from build123d import *

# Parameters (mm, degrees)
SKETCH1_W           = 20
SKETCH1_H           = 20
BOSS_EXTRUDE1_DEPTH = 5.4
SKETCH2_R           = 8
CUT_EXTRUDE1_DEPTH  = 5
SKETCH4_W           = 1
SKETCH4_H           = 20
CUT_EXTRUDE3_DEPTH  = 10
SKETCH3_R           = 1.5
CUT_EXTRUDE2_DEPTH  = 0.25
SKETCH5_W           = 5.4
SKETCH5_H           = 1
CUT_EXTRUDE4_DEPTH  = 0.25
FILLET1_R           = 1
CHAMFER1_SIZE       = 0.5


with BuildPart() as part:
    # Sketch1 → Boss-Extrude1 (new body)
    with BuildSketch(Plane.XY):
        Rectangle(SKETCH1_W, SKETCH1_H)
    extrude(amount=BOSS_EXTRUDE1_DEPTH)

    # Sketch2 → Cut-Extrude1 (cut)
    with BuildSketch(Plane.XY.offset(5.4)):
        Circle(SKETCH2_R)
    extrude(amount=-CUT_EXTRUDE1_DEPTH, mode=Mode.SUBTRACT)

    # Sketch4 → Cut-Extrude3 (cut)
    with BuildSketch(Plane.XY.offset(5.4)):
        with Locations((9.5, 0)):
            Rectangle(SKETCH4_W, SKETCH4_H)
    extrude(amount=-CUT_EXTRUDE3_DEPTH, mode=Mode.SUBTRACT)

    # Sketch3 → Cut-Extrude2 (cut)
    with BuildSketch(Plane(origin=(9, 0, 0), x_dir=(0, 0, -1), z_dir=(1, 0, 0))):
        with Locations(Location((-2.7, -5, 0), (0, 0, 90))):
            Circle(SKETCH3_R)
    extrude(amount=-CUT_EXTRUDE2_DEPTH, mode=Mode.SUBTRACT)

    # Sketch5 → Cut-Extrude4 (cut)
    with BuildSketch(Plane.ZY.offset(10)):
        with Locations((2.7, 5)):
            Rectangle(SKETCH5_W, SKETCH5_H)
    extrude(amount=-CUT_EXTRUDE4_DEPTH, mode=Mode.SUBTRACT)

    # Fillet1
    fillet1_edges = [part.edges().sort_by_distance(p)[0] for p in [
        (9, -10, 2.7),
        (9, 10, 2.7),
        (-10, -10, 2.7),
        (-10, 10, 2.7),
    ]]
    fillet(fillet1_edges, radius=FILLET1_R)

    # Chamfer1
    # the kernel refuses this chamfer: 0.5 mm, written as the material it takes off along each edge
    with BuildSketch(Plane(origin=(8, 10, 0), x_dir=(0, -0.9996219169112968, -0.02749587661058639), z_dir=(-1, 0, 0)), Plane(origin=(-9, -10, 5.4), x_dir=(0, -0.027495876610585647, -0.9996219169112968), z_dir=(1, 0, 0))) as chamfer1_piece_1:
        Polygon((CHAMFER1_SIZE * 0.999621916911, CHAMFER1_SIZE * 0.0274958766106), (-CHAMFER1_SIZE * 0.0274958766106, CHAMFER1_SIZE * 0.999621916911), (0, 0), align=None)
    extrude(amount=17, mode=Mode.SUBTRACT)
    with BuildSketch(Plane(origin=(-9, 9, 0), x_dir=(0, 1, 0), z_dir=(1, 0, 0))) as chamfer1_piece_2:
        Polygon((1 - CHAMFER1_SIZE, 0), (1, CHAMFER1_SIZE), (1, 0), align=None)
    revolve(axis=Axis((-9, 9, 0), (0, 0, 1)), revolution_arc=90, mode=Mode.SUBTRACT)
    with BuildSketch(Plane(origin=(-10, 5.785841494, 0), x_dir=(0.9996219169112968, 0, -0.02749587661058639), z_dir=(0, -1, 0))) as chamfer1_piece_3:
        Polygon((CHAMFER1_SIZE * 0.999621916911, CHAMFER1_SIZE * 0.0274958766106), (-CHAMFER1_SIZE * 0.0274958766106, CHAMFER1_SIZE * 0.999621916911), (0, 0), align=None)
    extrude(amount=14.785841494, mode=Mode.SUBTRACT)
    with BuildSketch(Plane(origin=(-10, 9, 0), x_dir=(0.9996219169112968, 0, -0.02749587661058639), z_dir=(0, -1, 0))) as chamfer1_piece_4:
        Polygon((CHAMFER1_SIZE * 0.999621916911, CHAMFER1_SIZE * 0.0274958766106), (-CHAMFER1_SIZE * 0.0274958766106, CHAMFER1_SIZE * 0.999621916911), (0, 0), align=None)
    extrude(amount=4.785841494, mode=Mode.SUBTRACT)
    with BuildSketch(Plane(origin=(-9, -9, 0), x_dir=(0, -1, 0), z_dir=(1, 0, 0))) as chamfer1_piece_5:
        Polygon((1 - CHAMFER1_SIZE, 0), (1, -CHAMFER1_SIZE), (1, 0), align=None)
    revolve(axis=Axis((-9, -9, 0), (0, 0, -1)), revolution_arc=90, mode=Mode.SUBTRACT)
    with BuildSketch(Plane(origin=(-9, -10, 0), x_dir=(0, -0.02749587661058563, 0.9996219169112968), z_dir=(1, 0, 0)), Plane(origin=(8, 10, 5.4), x_dir=(0, -0.9996219169112968, 0.027495876610585647), z_dir=(-1, 0, 0))) as chamfer1_piece_6:
        Polygon((CHAMFER1_SIZE * 0.999621916911, -CHAMFER1_SIZE * 0.0274958766106), (-CHAMFER1_SIZE * 0.0274958766106, -CHAMFER1_SIZE * 0.999621916911), (0, 0), align=None)
    extrude(amount=17, mode=Mode.SUBTRACT)
    with BuildSketch(Plane(origin=(-9, -9, 5.4), x_dir=(0, -1, 0), z_dir=(1, 0, 0))) as chamfer1_piece_7:
        Polygon((1, CHAMFER1_SIZE), (1 - CHAMFER1_SIZE, 0), (1, 0), align=None)
    revolve(axis=Axis((-9, -9, 5.4), (0, 0, -1)), revolution_arc=90, mode=Mode.SUBTRACT)
    with BuildSketch(Plane(origin=(-10, 9, 5.4), x_dir=(0.9996219169112968, 0, 0.027495876610585647), z_dir=(0, -1, 0))) as chamfer1_piece_8:
        Polygon((CHAMFER1_SIZE * 0.999621916911, -CHAMFER1_SIZE * 0.0274958766106), (-CHAMFER1_SIZE * 0.0274958766106, -CHAMFER1_SIZE * 0.999621916911), (0, 0), align=None)
    extrude(amount=4.785841494, mode=Mode.SUBTRACT)
    with BuildSketch(Plane(origin=(-10, 5.785841494, 5.4), x_dir=(0.9996219169112968, 0, 0.027495876610585647), z_dir=(0, -1, 0))) as chamfer1_piece_9:
        Polygon((CHAMFER1_SIZE * 0.999621916911, -CHAMFER1_SIZE * 0.0274958766106), (-CHAMFER1_SIZE * 0.0274958766106, -CHAMFER1_SIZE * 0.999621916911), (0, 0), align=None)
    extrude(amount=14.785841494, mode=Mode.SUBTRACT)
    with BuildSketch(Plane(origin=(-9, 9, 5.4), x_dir=(0, 1, 0), z_dir=(1, 0, 0))) as chamfer1_piece_10:
        Polygon((1 - CHAMFER1_SIZE, 0), (1, -CHAMFER1_SIZE), (1, 0), align=None)
    revolve(axis=Axis((-9, 9, 5.4), (0, 0, 1)), revolution_arc=90, mode=Mode.SUBTRACT)
    with BuildSketch(Plane(origin=(0, 0, 5.4), x_dir=(1, 0, 0), z_dir=(0, -1, 0))) as chamfer1_piece_11:
        Polygon((8 + CHAMFER1_SIZE, 0), (8, -CHAMFER1_SIZE), (8, 0), align=None)
    revolve(axis=Axis((0, 0, 5.4), (0, 0, 1)), mode=Mode.SUBTRACT)
    with BuildSketch(Plane(origin=(9, 9, 0), x_dir=(-0.9996219169112968, 0, -0.02749587661058639), z_dir=(0, -1, 0))) as chamfer1_piece_12:
        Polygon((CHAMFER1_SIZE * 0.999621916911, -CHAMFER1_SIZE * 0.0274958766106), (-CHAMFER1_SIZE * 0.0274958766106, -CHAMFER1_SIZE * 0.999621916911), (0, 0), align=None)
    extrude(amount=18, mode=Mode.SUBTRACT)
    with BuildSketch(Plane(origin=(9, 9, 5.4), x_dir=(-0.9996219169112968, 0, 0.027495876610585647), z_dir=(0, -1, 0))) as chamfer1_piece_13:
        Polygon((CHAMFER1_SIZE * 0.999621916911, CHAMFER1_SIZE * 0.0274958766106), (-CHAMFER1_SIZE * 0.0274958766106, CHAMFER1_SIZE * 0.999621916911), (0, 0), align=None)
    extrude(amount=18, mode=Mode.SUBTRACT)
    with BuildSketch(Plane(origin=(8, 9, 0), x_dir=(1, 0, 0), z_dir=(0, -1, 0))) as chamfer1_piece_14:
        Polygon((1 - CHAMFER1_SIZE, 0), (1, CHAMFER1_SIZE), (1, 0), align=None)
    revolve(axis=Axis((8, 9, 0), (0, 0, 1)), revolution_arc=90, mode=Mode.SUBTRACT)
    with BuildSketch(Plane(origin=(8, -9, 0), x_dir=(0, -1, 0), z_dir=(-1, 0, 0))) as chamfer1_piece_15:
        Polygon((1 - CHAMFER1_SIZE, 0), (1, CHAMFER1_SIZE), (1, 0), align=None)
    revolve(axis=Axis((8, -9, 0), (0, 0, 1)), revolution_arc=90, mode=Mode.SUBTRACT)
    with BuildSketch(Plane(origin=(8, 9, 5.4), x_dir=(1, 0, 0), z_dir=(0, -1, 0))) as chamfer1_piece_16:
        Polygon((1 - CHAMFER1_SIZE, 0), (1, -CHAMFER1_SIZE), (1, 0), align=None)
    revolve(axis=Axis((8, 9, 5.4), (0, 0, 1)), revolution_arc=90, mode=Mode.SUBTRACT)
    with BuildSketch(Plane(origin=(8, -9, 5.4), x_dir=(0, -1, 0), z_dir=(-1, 0, 0))) as chamfer1_piece_17:
        Polygon((1, -CHAMFER1_SIZE), (1 - CHAMFER1_SIZE, 0), (1, 0), align=None)
    revolve(axis=Axis((8, -9, 5.4), (0, 0, 1)), revolution_arc=90, mode=Mode.SUBTRACT)


solid = part.part
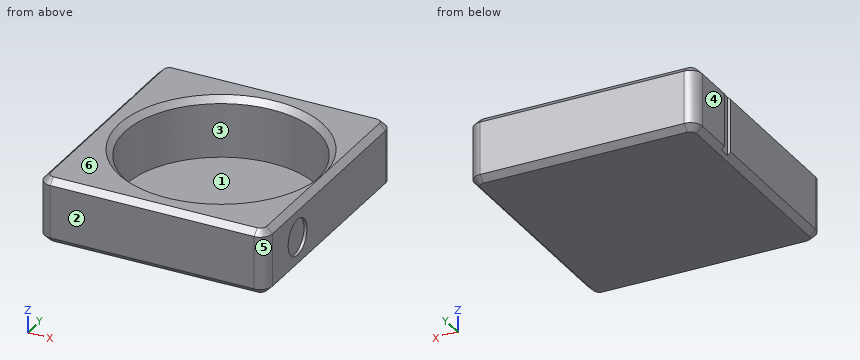
For this review, take the finished solid that the model builds, in its own axes (mm). Face numbers are marked on the shaded views. A direction names the side the tool comes from. Round coordinates to 2 decimals unless told otherwise and drop trailing zeros. Order: outer loops, then holes, each group sorted by start corner. A loop starts at its lowest first (then second) coordinate and runs counter-clockwise, first axis right, second up. Notation, with made-up numbers: (-1.5, -19) -> (17.5, -19) arc R36 cw to (17.5, 17) -> close; hole circle Ø6 at (71, 36). An arc over 180 degrees is marked (long way). Put each result on its own line as item: value.
Q1. Machinability: for the marked faces 1 and 2, which of the approach directions +Z, -Z, +X, -X, +Y, -Y give a long, thin tool a straight path to every point of the face, cutting with its end or side? Answer none if there is none.
Check result:
face 1: +Z
face 2: +Z, -Z, +X, -X, -Y
Q2. Add section B-B on x = 0. Write out the cut boundary in (y, z).
Check result:
outline: (-10, 0.5) -> (-9.5, 0) -> (9.5, 0) -> (10, 0.5) -> (10, 4.9) -> (9.5, 5.4) -> (8.5, 5.4) -> (8, 4.9) -> (8, 0.4) -> (-8, 0.4) -> (-8, 4.9) -> (-8.5, 5.4) -> (-9.5, 5.4) -> (-10, 4.9) -> close
Q3. Insertion check: pin 1 Ø5 at (x, y) = (3, 1) entering from +Z; pin 2 Ø0.8 at (y, z) = (5, 3) entering from -X; pin 3 Ø0.9 at (y, z) = (-5.5, 3) entering from +X. Each pin has a flat end and moves straight along its axis. Give the tip position at first contact, or say it passes through.
Check result:
pin 1: z = 0.4
pin 2: x = -9.75
pin 3: x = 8.75
Q4. For probe 1 along Y at (x, z) = (0, 2.75); probe 2 along Y at (x, z) = (-7, 0.55); probe 3 along Z at (x, y) = (5, 0.25), list the stretches that pass through material, from the lowest coordinate up. Write a range as [from, to].
Check result:
probe 1: [-10, -8], [8, 10]
probe 2: [-10, -3.87], [3.87, 10]
probe 3: [0, 0.4]
Q5. Add section C-C on z = 3.05. Write out the cut boundary in (x, y), plus the area to 3 significant figures.
Check result:
outline: (-10, -9) arc R1 ccw to (-9, -10) -> (8, -10) arc R1 ccw to (9, -9) -> (9, -6.46) -> (8.75, -6.46) -> (8.75, -3.54) -> (9, -3.54) -> (9, 9) arc R1 ccw to (8, 10) -> (-9, 10) arc R1 ccw to (-10, 9) -> (-10, 5.5) -> (-9.75, 5.5) -> (-9.75, 4.5) -> (-10, 4.5) -> close; hole circle Ø16 at (0, 0)
area: 177 mm2
Q6. Mouldability with a two-part tool opening along X and no side actions: class the marked faces 3, 4, 5 and 6 as pulls with the +X half, pulls with the -X half, needs draft (parallel to the pull), parting line crosses it, or undercut.
Check result:
face 3: undercut
face 4: pulls with the -X half
face 5: pulls with the +X half
face 6: needs draft
Q7. Add section A-A on z = 0.75. Write out the cut boundary in (x, y).
Check result:
outline: (-10, -9) arc R1 ccw to (-9, -10) -> (8, -10) arc R1 ccw to (9, -9) -> (9, 9) arc R1 ccw to (8, 10) -> (-9, 10) arc R1 ccw to (-10, 9) -> (-10, 5.5) -> (-9.75, 5.5) -> (-9.75, 4.5) -> (-10, 4.5) -> close; hole circle Ø16 at (0, 0)
